Geometry check sheet. Reference: drawing and pictorial views, mm from the part's lowest x, y, z. A direction names the side the tool comes from. Give positions to 0.01 mm unless a question says otherwise; leave off trailing zeros. Loops run counter-clockwise (first coordinate to the right, second up) from the corner with the lowest first, then second, coordinate; pieces in that order, holes last. Notation, with made-up numbers: (40.5, -9) -> (57.5, -9) arc R25 cw to (57.5, 5) -> close; hole circle Ø9 at (64.25, 54.25). An arc over 180 degrees is marked (long way). Answer in a Markdown table with one row per item. Add a question column.
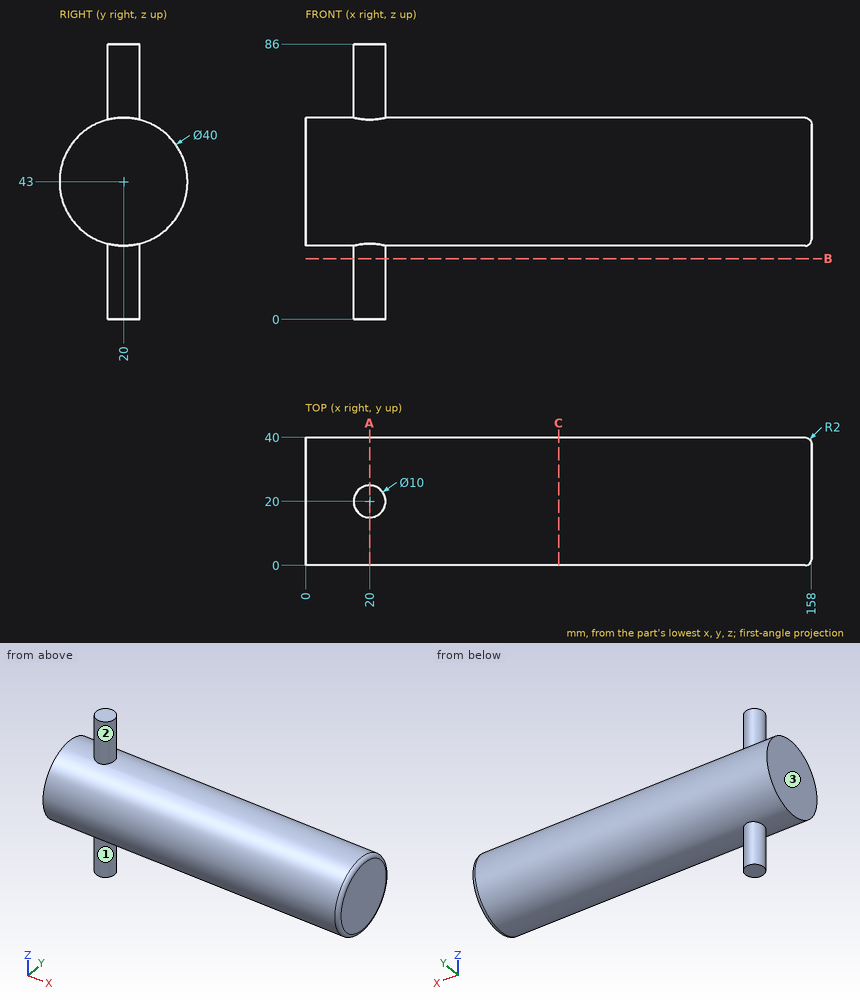
1. Sectioned sample at B-B (z = 19). Enter the section's corners in (x, y), plus the area to 3 significant figures.
2. Material ranges on L1, parallel to Z at x = 54.5, y = 20.5; L2, parallel to Y at x = 7.5, z = 38.5; L3, parallel to Y at x = 116, z = 52.5, recorded low to high. Write a range as from..to.
3. Sectioned sample at C-C (x = 79). Enter the section's corners in (y, z), plus the area to 3 significant figures.
4. Gauge pin test, flat ends, axial feed: pin 1 Ø1 at (y, z) = (23, 66.5) entering from +X; pin 2 Ø10 at (x, z) = (90, 33.5) entering from +Y; pin 3 Ø1 at (x, y) = (114, 24.5) entering from -Z. Record the tip position at first contact, or that the pin passes through.
5. Access from +Z, -Z, +X, -X, +Y, -Y to the whole of each face (thin tool, end or side, straight path). Record for the marked faces 1, 2 and 3.
6. Sectioned sample at A-A (x = 20). Enter the section's corners in (y, z).
Response:
| question | item | result |
|---|---|---|
| 1 | outline | circle Ø10 at (20, 20) |
| 1 | area | 78.5 mm2 |
| 2 | L1 | z = 23.01..62.99 |
| 2 | L2 | y = 0.51..39.49 |
| 2 | L3 | y = 2.4..37.6 |
| 3 | outline | circle Ø40 at (20, 43) |
| 3 | area | 1,260 mm2 |
| 4 | pin 1 | stops at x = 24.33 |
| 4 | pin 2 | stops at y = 39.49 |
| 4 | pin 3 | stops at z = 23.4 |
| 5 | face 1 | -Z |
| 5 | face 2 | +Z |
| 5 | face 3 | +Z, -Z, -X, +Y, -Y |
| 6 | outline | (15, 0) -> (25, 0) -> (25, 23.64) arc R20 ccw to (25, 62.36) -> (25, 86) -> (15, 86) -> (15, 62.36) arc R20 ccw to (15, 23.64) -> close |
